The listing builds one solid part. Answer for the finished solid, in the listing's coordinates (mm). A direction names the side the tool comes from. Give positions to 0.01 mm unless a question says otherwise; leave off trailing zeros. Order: outer loops, then holes, each group sorted by start corner. A loop starts at its lowest first (then second) coordinate and runs counter-clockwise, first axis right, second up.
```python
from build123d import *

# Parameters (mm, degrees)
CYLINDER098_R     = 15
CYLINDER098_DEPTH = 4
BOX249_W          = 2
BOX249_H          = 10
BOX249_DEPTH      = 9
BOX250_W          = 2
BOX250_H          = 4
BOX250_DEPTH      = 13
BOX251_W          = 2
BOX251_H          = 14
BOX251_DEPTH      = 3
FILLET064_R       = 1.5


with BuildPart() as cylinder178:
    # Cylinder098 → Cylinder098 (new body)
    with BuildSketch(Plane(origin=(117, 31, -15), x_dir=(0, 0, -1), z_dir=(1, 0, 0))):
        Circle(CYLINDER098_R)
    extrude(amount=CYLINDER098_DEPTH)


with BuildPart() as cut130:
    # Box249 → Box249 (new body)
    with BuildSketch(Plane(origin=(118, 40, -15), x_dir=(1, 0, 0), z_dir=(0, 0, 1))):
        with Locations((1, 5)):
            Rectangle(BOX249_W, BOX249_H)
    extrude(amount=BOX249_DEPTH)

    # Cut130: cut Cylinder178
    add(cylinder178.part, mode=Mode.SUBTRACT)


with BuildPart() as cube238:
    # Box250 → Box250 (new body)
    with BuildSketch(Plane(origin=(118, 46, -28), x_dir=(1, 0, 0), z_dir=(0, 0, 1))):
        with Locations((1, 2)):
            Rectangle(BOX250_W, BOX250_H)
    extrude(amount=BOX250_DEPTH)


with BuildPart() as fillet064:
    # Box251 → Box251 (new body)
    with BuildSketch(Plane(origin=(118, 36, -6), x_dir=(1, 0, 0), z_dir=(0, 0, 1))):
        with Locations((1, 7)):
            Rectangle(BOX251_W, BOX251_H)
    extrude(amount=BOX251_DEPTH)

    # Fusion078: union Cut130, Cube238
    add(cut130.part)
    add(cube238.part)

    # Fillet064
    fillet064_edges = [fillet064.edges().sort_by_distance(p)[0] for p in [
        (120, 36, -4.5),
        (120, 48, -28),
    ]]
    fillet(fillet064_edges, radius=FILLET064_R)


solid = fillet064.part
```
1) Find section C-C (z = -23.25). Write down the section's boundary in (x, y), then the cut area to 3 significant figures.
Geometry says:
outline: (118, 46) - (120, 46) - (120, 50) - (118, 50) - close
area: 8.00 mm2
2) Straight lines are drawn through the part: probe 1 along Z at (x, y) = (118.5, 38); probe 2 along Y at (x, z) = (119.3, -20); probe 3 along Z at (x, y) = (118.6, 49.25). For each, find the intervals that lie inside material, in ascending order.
Geometry says:
probe 1: z = -6 to -3
probe 2: y = 46 to 50
probe 3: z = -28 to -3
3) Find section A-A (x = 119.7). Write down the section's boundary in (y, z).
Geometry says:
outline: (36.6, -6) - (43, -6) arc R15 cw to (46, -15) - (46, -27.4) - (50, -27.4) - (50, -3) - (36.6, -3) - close
4) Given P1, Ø1, axis at x = 119, z = -19, coming from the -Y side, flat-ended and moving along its own axis, determine where the tip first touches the part or whether it passes through.
Geometry says:
P1: stops at y = 46
5) A tool of negligible diameter and unlimited length cuts with its end or side. For faces 1 (the flat face through (119, 46, -22)), 2 (the flat face through (118, 46.01, -12.9)), from which of +Z, -Z, +X, -X, +Y, -Y can it reach the whole face along a straight path? Write none if from no direction.
Geometry says:
face 1: -Z, +X, -X, -Y
face 2: +Z, -Z, -X, +Y, -Y
6) Find section B-B (y = 39.75). Write down the section's boundary in (x, z), then the cut area to 3 significant figures.
Geometry says:
outline: (118, -6) - (120, -6) - (120, -3) - (118, -3) - close
area: 6.00 mm2
